For this review, take the finished solid that the model builds, in its own axes (mm). A direction names the side the tool comes from. Give positions to 0.01 mm unless a question says otherwise; leave off trailing zeros. Loops run counter-clockwise (first coordinate to the right, second up) from the corner with the lowest first, then second, coordinate; pieces in that order, holes last.
```python
from build123d import *

# Parameters (mm, degrees)
F1_DEPTH = 25.4
F2_W     = 12.2484653257
F2_H     = 6.995950315
F3_DEPTH = 25.4
F4_W     = 12.7
F4_H     = 6.35
F5_DEPTH = 25.4


with BuildPart() as f1:
    # F0 (on Front) → F1 (new body)
    with BuildSketch(Plane.XZ):
        Polygon((-58.1661015928, 43.1416464728), (-58.0037304439, 11.3920616628), (-45.3037304439, 11.3920616628), (-45.3037304439, 17.7420616628), (-32.6037304439, 17.7420616628), (-33.1024721118, 11.411678045), (-20.4096810303, 10.9838292846), (-20.0683039551, 42.7319939826), align=None)
    extrude(amount=F1_DEPTH)

    # F2 (on face) → F3 (cut)
    with BuildSketch(Plane(origin=(-57.9439546086, 0, -0.2963322682), x_dir=(0, -1, 0), z_dir=(-0.9999869232, 0, -0.0051140519))):
        with Locations((12.7056662459, 39.9405716228)):
            Rectangle(F2_W, F2_H)
    extrude(amount=-F3_DEPTH, mode=Mode.SUBTRACT)

    # F4 (on face) → F5 (cut)
    with BuildSketch(Plane(origin=(-20.5254132218, 0, 0.2207026957), x_dir=(0, 1, 0), z_dir=(0.9999421952, 0, -0.0107520339))):
        with Locations((-12.7976922482, 39.338748785)):
            Rectangle(F4_W, F4_H)
    extrude(amount=-F5_DEPTH, mode=Mode.SUBTRACT)


solid = f1.part
```
Q1. Machinability: for faces 1 (the flat face through (-39, 0, 27)), 2 (the flat face through (-45.304, -13, 15)), 3 (the flat face through (-52, -13, 11.392)), 4 (the flat face through (-33, -6.448, 40)), 5 (the flat face through (-32.85, -12.52, 14.62)), which of the approach directions +Z, -Z, +X, -X, +Y, -Y give a long, thin tool a straight path to every point of the face, cutting with its end or side? Answer none if there is none.
Answers:
face 1: +Z, -Z, +X, -X, +Y
face 2: -Z, +Y, -Y
face 3: -Z, -X, +Y, -Y
face 4: +Z, +X
face 5: +Y, -Y
Q2. For pin 1 Ø6.5 at (x, y) = (-54, -8.5) entering from -Z; pin 2 Ø14 at (x, y) = (-37.5, -13) entering from -Z; pin 3 Ø2 at (x, y) = (-40.5, -9.5) entering from -Z, all flat-tipped, find the tip position at first contact; note any pin that passes through.
Answers:
pin 1: stops at z = 11.39
pin 2: stops at z = 11.32
pin 3: stops at z = 17.74
Q3. Consider section C-C on x = -44. Give the boundary of the cut face in (y, z).
Answers:
outline: (-25.4, 17.74) - (0, 17.74) - (0, 42.99) - (-6.45, 42.99) - (-6.45, 36.64) - (-6.58, 36.64) - (-6.58, 36.22) - (-18.83, 36.22) - (-18.83, 36.64) - (-19.15, 36.64) - (-19.15, 42.99) - (-25.4, 42.99) - close
Q4. For probe 1 along Y at (x, z) = (-40, 40); probe 2 along X at (y, z) = (-18.75, 16.5); probe 3 along X at (y, z) = (-5.75, 42.5), list the stretches that pass through material, from the lowest coordinate up.
Answers:
probe 1: y = -25.4 to -19.15, -6.45 to 0
probe 2: x = -58.03 to -45.3, -32.7 to -20.35
probe 3: x = -58.16 to -20.07
Q5. Consider section A-A on z = 13. Give the boundary of the cut face in (x, y).
Answers:
outline: (-58.01, -25.4) - (-45.3, -25.4) - (-45.3, 0) - (-58.01, 0) - close; (-32.98, -25.4) - (-20.39, -25.4) - (-20.39, 0) - (-32.98, 0) - close
Q6. Consider section D-D on z = 17. Give the boundary of the cut face in (x, y) (3 decimals).
Answers:
outline: (-58.032, -25.4) - (-45.304, -25.4) - (-45.304, 0) - (-58.032, 0) - close; (-32.662, -25.4) - (-20.345, -25.4) - (-20.345, 0) - (-32.662, 0) - close
Q7. Mouldability with a two-part tool opening along Y and no side actions: class faces 6 (the flat face through (-39, -25.4, 27)), 7 (the flat face through (-39, -13, 17.742)), 8 (the flat face through (-51, -18.83, 40)) as +Y half, -Y half, draft (parallel to the pull), parting line (faces both ways), or undercut.
Answers:
face 6: -Y half
face 7: draft
face 8: undercut
Q8. Consider section B-B on y = -9. Give the boundary of the cut face in (x, z).
Answers:
outline: (-58.13, 36.15) - (-58, 11.39) - (-45.3, 11.39) - (-45.3, 17.74) - (-32.6, 17.74) - (-33.1, 11.41) - (-20.41, 10.98) - (-20.14, 36.38) - (-32.73, 36.52) - (-32.73, 36.28) - close
